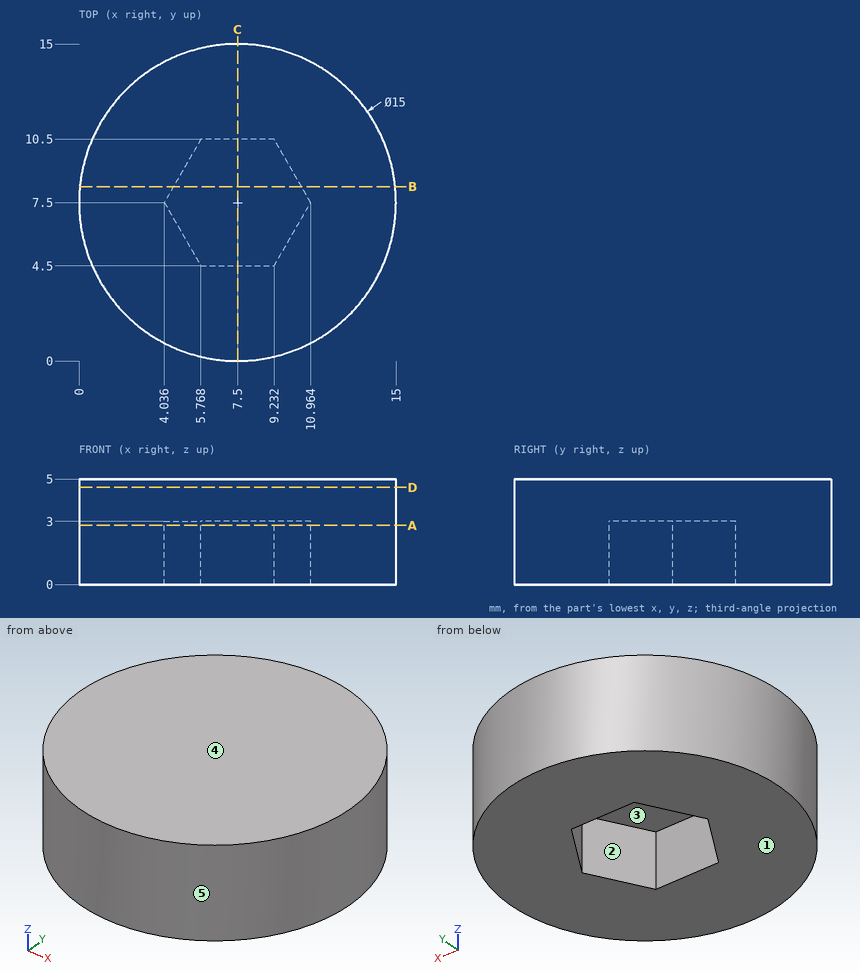
Design review of the part shown in the three views and the two pictorial views. Dimensions are in mm from the part's minimum x, y and z. A direction names the side the tool comes from. Coordinates: 2 decimals unless noted, no trailing zeros. Write each loop counter-clockwise with the first axis right and the second up, starting at its lowest first coordinate (ties: lowest second). Pieces come first, ordered by that corner, then holes.
(1) Tool access review of the marked faces 1 and 2: name each direction out of +Z, -Z, +X, -X, +Y, -Y from which nothing blocks a thin tool from reaching the whole face with its end or side.
(2) The part is to be moulded in two halves that separate along X. For the marked faces 3, 4 and 5, say which applies: +X half, -X half, draft (parallel to the pull), parting line (faces both ways), or undercut.
(3) Add section D-D on z = 4.6. Give the boundary of the cut face in (x, y).
(4) Wall thickness on probe 1 along Y at (x, z) = (5.75, 0.35); probe 2 along X at (y, z) = (7.25, 3.5); probe 3 along X at (y, z) = (8.25, 1.1): over which ranges is each line inside the solid? List them lowest first.
(5) Add section A-A on z = 2.8. Give the boundary of the cut face in (x, y), then the cut area to 3 significant figures.
(6) Add section C-C on x = 7.5. Give the boundary of the cut face in (y, z).
(7) For pin 1 Ø2 at (y, z) = (3, 2.5) entering from +X; pin 2 Ø1 at (x, z) = (5, 3) entering from +Y; pin 3 Ø5 at (x, y) = (8, 6.5) entering from -Z; pin 4 Ø1 at (y, z) = (2, 3.5) entering from -X, all flat-tipped, find the tip position at first contact; note any pin that passes through.
(8) Add section B-B on y = 8.25. Give the boundary of the cut face in (x, z).
Answer sheet:
1. face 1: -Z, +X, -X, +Y, -Y
1. face 2: -Z
2. face 3: undercut
2. face 4: draft
2. face 5: parting line
3. outline: circle Ø15 at (7.5, 7.5)
4. probe 1: y = 0.21 to 4.53, 10.47 to 14.79
4. probe 2: x = 0 to 15
4. probe 3: x = 0.04 to 4.47, 10.53 to 14.96
5. outline: circle Ø15 at (7.5, 7.5); hole (4.04, 7.5) - (5.77, 4.5) - (9.23, 4.5) - (10.96, 7.5) - (9.23, 10.5) - (5.77, 10.5) - close
5. area: 146 mm2
6. outline: (0, 0) - (4.5, 0) - (4.5, 3) - (10.5, 3) - (10.5, 0) - (15, 0) - (15, 5) - (0, 5) - close
7. pin 1: stops at x = 14.13
7. pin 2: stops at y = 14.73
7. pin 3: stops at z = 0
7. pin 4: stops at x = 1.91
8. outline: (0.04, 0) - (4.47, 0) - (4.47, 3) - (10.53, 3) - (10.53, 0) - (14.96, 0) - (14.96, 5) - (0.04, 5) - close
